Verification items for the finished model (mm, model axes). A direction names the side the tool comes from. Give positions to 0.01 mm unless a question says otherwise; leave off trailing zeros. Write each loop counter-clockwise with the first axis right and the second up, starting at its lowest first coordinate (ties: lowest second). Pieces come first, ordered by that corner, then holes. Notation, with made-up numbers: (47, 38.25) -> (88, 38.25) arc R22 cw to (88, 44.25) -> close; hole circle Ø3 at (40, -31.75). An arc over 180 degrees is marked (long way). Answer as CSV lines item,"result".
```python
from build123d import *

# Parameters (mm, degrees)
SKETCH1_W                   = 25.4
SKETCH1_H                   = 76.2
BOSS_EXTRUDE1_DEPTH         = 6.35
BOSS_EXTRUDE2_DEPTH         = 6.35
F_1_4_START                 = 19.05
F_1_4_CLEARANCE_SLOT1_DEPTH = 6.35
F_1_4_CLEARANCE_HOLE1_D     = 6.7564


# Read off the part's stored shape, not the designer's step: 1/4 Clearance Slot1
with BuildPart() as part:
    # Sketch1 → Boss-Extrude1 (new body)
    with BuildSketch(Plane.XY):
        with Locations((12.7, 38.1)):
            Rectangle(SKETCH1_W, SKETCH1_H)
    extrude(amount=BOSS_EXTRUDE1_DEPTH)

    # Sketch2 → Boss-Extrude2 (add)
    with BuildSketch(Plane(origin=(25.4, 0, 0), x_dir=(0, 0, -1), z_dir=(1, 0, 0))):
        Polygon((-6.35, 76.2), (-6.35, 0), (-20.909871939, 0), (-25.4, 4.490128061), (-25.4, 71.709871939), (-20.909871939, 76.2), align=None)
    extrude(amount=-BOSS_EXTRUDE2_DEPTH)

    # 1/4 Clearance Slot1 outline → 1/4 Clearance Slot1 (cut)
    with BuildSketch(Plane.YZ.offset(F_1_4_START)):
        with BuildLine():
            ThreePointArc((22.4282, 18.8468), (19.05, 22.225), (15.6718, 18.8468))
            Line((15.6718, 18.8468), (15.6718, 12.9032))
            ThreePointArc((15.6718, 12.9032), (19.05, 9.525), (22.4282, 12.9032))
            Line((22.4282, 12.9032), (22.4282, 18.8468))
        make_face()
        with BuildLine():
            ThreePointArc((60.5282, 18.8468), (57.15, 22.225), (53.7718, 18.8468))
            Line((53.7718, 18.8468), (53.7718, 12.9032))
            ThreePointArc((53.7718, 12.9032), (57.15, 9.525), (60.5282, 12.9032))
            Line((60.5282, 12.9032), (60.5282, 18.8468))
        make_face()
    extrude(amount=F_1_4_CLEARANCE_SLOT1_DEPTH, mode=Mode.SUBTRACT)

    # 1/4 Clearance Hole1 (through all)
    with Locations(Plane.XY.offset(6.35)):
        with Locations((9.525, 63.5), (9.525, 12.7)):
            Hole(F_1_4_CLEARANCE_HOLE1_D / 2)


solid = part.part
```
1) Section check A-A (y = 63.5). Record the boundary of the cut face in (x, z).
Reported:
outline,"(0, 0) -> (6.15, 0) -> (6.15, 6.35) -> (0, 6.35) -> close; (12.9, 0) -> (25.4, 0) -> (25.4, 25.4) -> (19.05, 25.4) -> (19.05, 6.35) -> (12.9, 6.35) -> close"
2) Section check B-B (z = 17.25). Record the boundary of the cut face in (x, y).
Reported:
outline,"(19.05, 0) -> (25.4, 0) -> (25.4, 15.67) -> (19.05, 15.67) -> close; (19.05, 22.43) -> (25.4, 22.43) -> (25.4, 53.77) -> (19.05, 53.77) -> close; (19.05, 60.53) -> (25.4, 60.53) -> (25.4, 76.2) -> (19.05, 76.2) -> close"
3) Depth check by flat-ended pin: pin 1 (5 mm diameter, centred on x = 14, y = 46.5, fed in from +Z); pin 2 (8 mm diameter, centred on x = 9.525, y = 63.5, fed in from -Z); pin 3 (4 mm diameter, centred on x = 9.525, y = 12.7, fed in from -Z). Enter the tip coordinate at first touch or a pass-through.
Reported:
pin 1,"z = 6.35"
pin 2,"z = 0"
pin 3,"through"
4) Section check C-C (x = 12). Record the boundary of the cut face in (y, z).
Reported:
outline,"(0, 0) -> (10.4, 0) -> (10.4, 6.35) -> (0, 6.35) -> close; (15, 0) -> (61.2, 0) -> (61.2, 6.35) -> (15, 6.35) -> close; (65.8, 0) -> (76.2, 0) -> (76.2, 6.35) -> (65.8, 6.35) -> close"
5) Section check D-D (y = 19.05). Record the boundary of the cut face in (x, z) (3 decimals), and give its area (3 significant figures).
Reported:
outline,"(0, 0) -> (25.4, 0) -> (25.4, 9.525) -> (19.05, 9.525) -> (19.05, 6.35) -> (0, 6.35) -> close; (19.05, 22.225) -> (25.4, 22.225) -> (25.4, 25.4) -> (19.05, 25.4) -> close"
area,"202 mm²"
6) Tool access check on faces 1 (the flat face through (22.27, 2.21, 23.12)), 2 (the flat face through (9, 39, 6.35)), 3 (the flat face through (22, 53.772, 16)). Record the directions out of +Z, -Z, +X, -X, +Y, -Y that give a thin tool (end or side, any length) a straight path to the whole face; none if there is none.
Reported:
face 1,"+Z, +X, -X, -Y"
face 2,"+Z, -X, +Y, -Y"
face 3,"+X, -X"
7) Scan lines: line 1 along Y through (x, z) = (10.5, 2.5); line 2 along X through (y, z) = (26.5, 14.5); line 3 along Z through (x, y) = (6.25, 66). Record each from-to range of solid material in increasing order.
Reported:
line 1,"0 to 9.47, 15.93 to 60.27, 66.73 to 76.2"
line 2,"19.05 to 25.4"
line 3,"0 to 6.35"
8) Draft check along Y on faces 4 (the flat face through (22, 60.528, 16)), 5 (the flat face through (16, 76.2, 6)), 6 (the flat face through (19.05, 39, 16)). Enter one of: +Y half, -Y half, draft (parallel to the pull), parting line (faces both ways), or undercut.
Reported:
face 4,"undercut"
face 5,"+Y half"
face 6,"draft"
